The listing builds one solid part. Answer for the finished solid, in the listing's coordinates (mm). Face numbers are marked on the shaded views. A direction names the side the tool comes from. Give positions to 0.01 mm unless a question says otherwise; leave off trailing zeros. Loops run counter-clockwise (first coordinate to the right, second up) from the corner with the lowest first, then second, coordinate; pieces in that order, holes last. Notation, with made-up numbers: (82.25, -31) - (117.25, -31) arc R27 ccw to (117.25, 1) - close; hole circle Ø2 at (26.5, 5). An arc over 180 degrees is marked (long way). Answer as CSV lines item,"result". Start each with the question number.
1) A cutting plane is placed at A-A (x = 11.25). Determine the outline of the cut face in (y, z).
2) A cutting plane is placed at C-C (z = -31). Determine the outline of the cut face in (x, y), and give its area (3 significant figures).
3) Find the intervals of material crossed by line 1 along Y through (x, z) = (1, -45.5); line 2 along Z through (x, y) = (-4.5, 46); line 3 along Z through (x, y) = (7, 72), in increasing order.
4) A cutting plane is placed at B-B (y = 28.5). Determine the outline of the cut face in (x, z).
5) Flat-ended cylindrical pins translate along their axes: pin 1 (3 mm diameter, centred on x = -2, y = 56.5, fed in from -Z); pin 2 (8 mm diameter, centred on x = 8, z = -43, fed in from +Y). Find the tip coordinate at first contact, or state that the pin passes through.
6) For the marked faces 1 and 2, determine the directions among +Z, -Z, +X, -X, +Y, -Y from which every point of the face is accessible in a straight line to the end or side of a thin tool.
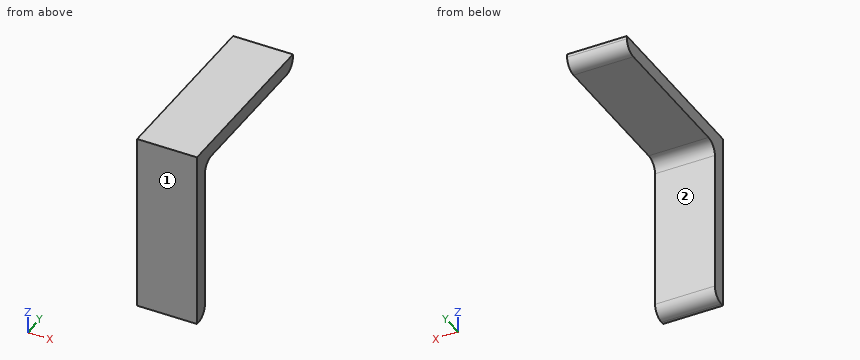
```python
from build123d import *

# Parameters (mm, degrees)
BOSS_EXTRUDE1_DEPTH      = 12.7
BOSS_EXTRUDE1_DEPTH_BACK = 12.7


with BuildPart() as part:
    # Sketch1 → Boss-Extrude1 (new, two sides: drawn at the far end of the back side and taken through both)
    with BuildSketch(Plane(origin=(0, 0, 0), x_dir=(0, 0, -1), z_dir=(1, 0, 0)).offset(-BOSS_EXTRUDE1_DEPTH_BACK)):
        with BuildLine():
            Line((0, 76.2), (0, 0))
            Line((0, 0), (76.2, 0))
            Line((76.2, 0), (76.2, 1.27))
            ThreePointArc((76.2, 1.27), (74.712102448, 4.862102448), (71.12, 6.35))
            Line((71.12, 6.35), (11.43, 6.35))
            ThreePointArc((11.43, 6.35), (7.837897552, 7.837897552), (6.35, 11.43))
            Line((6.35, 11.43), (6.35, 71.12))
            ThreePointArc((6.35, 71.12), (4.862102448, 74.712102448), (1.27, 76.2))
            Line((1.27, 76.2), (0, 76.2))
        make_face()
    extrude(amount=BOSS_EXTRUDE1_DEPTH + BOSS_EXTRUDE1_DEPTH_BACK)


solid = part.part
```
Ans:
1,outline,"(0, -76.2) - (1.27, -76.2) arc R5.08 ccw to (6.35, -71.12) - (6.35, -11.43) arc R5.08 cw to (11.43, -6.35) - (71.12, -6.35) arc R5.08 ccw to (76.2, -1.27) - (76.2, 0) - (0, 0) - close"
2,outline,"(-12.7, 0) - (12.7, 0) - (12.7, 6.35) - (-12.7, 6.35) - close"
2,area,"161 mm2"
3,line 1,"0 to 6.35"
3,line 2,"-6.35 to 0"
3,line 3,"-6.27 to 0"
4,outline,"(-12.7, -6.35) - (12.7, -6.35) - (12.7, 0) - (-12.7, 0) - close"
5,pin 1,"z = -6.35"
5,pin 2,"y = 6.35"
6,face 1,"+Z, -Z, +X, -X, -Y"
6,face 2,"-Z, +X, -X, +Y"
